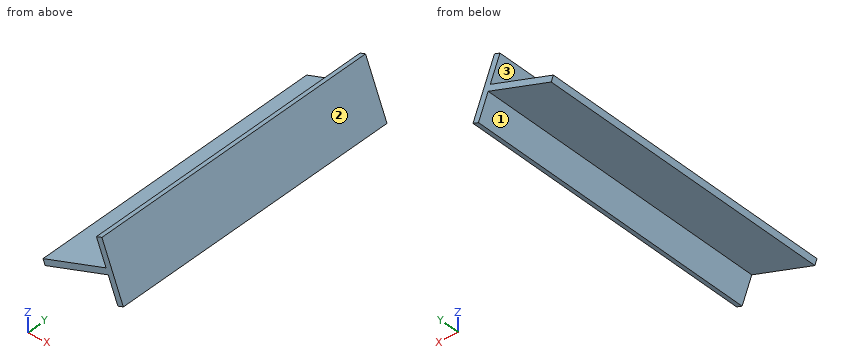
```python
from build123d import *

# Parameters (mm, degrees)
F1_DEPTH = 400


# Not quite as in the source:
# - the program builds the solid bodies; features that only make, move or delete a surface that nothing else refers to are left out


with BuildPart() as f1:
    # F0 (on Front) → F1 (new body)
    with BuildSketch(Plane.XZ):
        Polygon((-80.0059014217, 7.4499422376), (-77.090706633, 0), (8.5836290999, 33.5247400694), (21.7020056488, 0), (29.1519478864, 2.9151947886), (0, 77.4146171651), (-7.4499422376, 74.4994223765), (5.6684343113, 40.9746823071), align=None)
    extrude(amount=-F1_DEPTH)


solid = f1.part
```
Verification items for the finished model (mm, model axes). Face numbers are marked on the shaded views. Coordinates: 2 decimals unless noted, no trailing zeros. Loops run counter-clockwise (first coordinate to the right, second up) from the corner with the lowest first, then second, coordinate; pieces in that order, holes last. Notation, with made-up numbers: (85.25, 69) -> (111.25, 69) arc R30 ccw to (111.25, 107) -> close; hole circle Ø10 at (10.5, 76.25). An arc over 180 degrees is marked (long way). Answer in a Markdown table with one row per item. Add a question column.
1. Section check D-D, the plane z = 56. Enter the section's corners in (x, y), then the cut area to 3 significant figures.
2. Section check A-A, the plane z = 29. Enter the section's corners in (x, y), then the cut area to 3 significant figures.
3. Material ranges on probe 1 along Z at (x, y) = (-16.5, 255.5); probe 2 along X at (y, z) = (291, 59); probe 3 along X at (y, z) = (203.5, 63), recorded low to high. Write a range as [from, to].
4. Section check B-B, the plane y = 272.5. Enter the section's corners in (x, z), then the cut area to 3 significant figures.
5. Section check C-C, the plane x = -49. Enter the section's corners in (y, z).
6. Draft check along Z on the marked faces 1, 2 and 3. Enter one of: +Z half, -Z half, draft (parallel to the pull), parting line (faces both ways), or undercut.
7. Depth check by flat-ended pin: P1, Ø1, axis at x = -4, y = 85, coming from the -Z side; P2, Ø10, axis at x = -11, z = 65.5, coming from the +Y side; P3, Ø1.5, axis at x = -47.5, y = 291, coming from the +Z side; P4, Ø2, axis at x = -40, y = 278.5, coming from the +Z side. Enter the tip coordinate at first touch or a pass-through.
Derived:
| question | item | result |
|---|---|---|
| 1 | outline | (-0.21, 0) -> (8.38, 0) -> (8.38, 400) -> (-0.21, 400) -> close |
| 1 | area | 3,440 mm² |
| 2 | outline | (-24.93, 0) -> (-2.98, 0) -> (-2.98, 400) -> (-24.93, 400) -> close; (10.35, 0) -> (18.94, 0) -> (18.94, 400) -> (10.35, 400) -> close |
| 2 | area | 12,200 mm² |
| 3 | probe 1 | z = [23.71, 32.3] |
| 3 | probe 2 | x = [-1.38, 7.21] |
| 3 | probe 3 | x = [-2.95, 5.64] |
| 4 | outline | (-80.01, 7.45) -> (-77.09, 0) -> (8.58, 33.52) -> (21.7, 0) -> (29.15, 2.92) -> (0, 77.41) -> (-7.45, 74.5) -> (5.67, 40.97) -> close |
| 4 | area | 1,380 mm² |
| 5 | outline | (0, 10.99) -> (400, 10.99) -> (400, 19.58) -> (0, 19.58) -> close |
| 6 | face 1 | -Z half |
| 6 | face 2 | +Z half |
| 6 | face 3 | undercut |
| 7 | P1 | stops at z = 28.41 |
| 7 | P2 | passes through |
| 7 | P3 | stops at z = 20.46 |
| 7 | P4 | stops at z = 23.5 |
